```python
from build123d import *

# Parameters (mm, degrees)
SKETCH1_R               = 4.5
BOSS_EXTRUDE1_DEPTH     = 5
FILLET1_R               = 1
CUT_EXTRUDE1_DEPTH      = 78.139851996
CUT_EXTRUDE1_DEPTH_BACK = 78.139851996
CUT_EXTRUDE3_DEPTH      = 80.375373419
CUT_EXTRUDE3_DEPTH_BACK = 80.375373419


with BuildPart() as part:
    # Sketch1 → Boss-Extrude1 (new body)
    with BuildSketch(Plane.XY):
        with BuildLine():
            Line((-21.758850115, -29.16270467), (-30.758850115, -7.434782609))
            Line((-30.758850115, -7.434782609), (-30.758850115, 52.565217391))
            ThreePointArc((-30.758850115, 52.565217391), (-12.758850115, 70.565217391), (5.241149885, 52.565217391))
            Line((5.241149885, 52.565217391), (5.241149885, -7.434782609))
            Line((5.241149885, -7.434782609), (-3.758850115, -29.16270467))
            Line((-3.758850115, -29.16270467), (-12.758850115, -7.434782609))
            Line((-12.758850115, -7.434782609), (-21.758850115, -29.16270467))
        make_face()
        with Locations((-12.758850115, 52.565217391)):
            Circle(SKETCH1_R, mode=Mode.SUBTRACT)
    extrude(amount=BOSS_EXTRUDE1_DEPTH)

    # Fillet1
    fillet1_edges = [part.edges().sort_by_distance(p)[0] for p in [
        (5.241149885, 22.565217391, 5),
        (-17.258850115, 52.565217391, 0),
        (-17.258850115, 52.565217391, 5),
        (-12.758850115, 70.565217391, 5),
        (-30.758850115, 22.565217391, 5),
        (-30.758850115, 22.565217391, 0),
        (-12.758850115, 70.565217391, 0),
        (5.241149885, 22.565217391, 0),
    ]]
    fillet(fillet1_edges, radius=FILLET1_R)

    # Sketch5 → Cut-Extrude1 (cut, two sides: drawn at the far end of the back side and taken through both)
    with BuildSketch(Plane(origin=(0, 0, 0), x_dir=(0, 0, -1), z_dir=(1, 0, 0)).offset(-CUT_EXTRUDE1_DEPTH_BACK)):
        Polygon((-2.5, -29.16270467), (-5, -9.848996171), (-5, -29.16270467), align=None)
    extrude(amount=CUT_EXTRUDE1_DEPTH + CUT_EXTRUDE1_DEPTH_BACK, mode=Mode.SUBTRACT)

    # Sketch9 → Cut-Extrude3 (cut, two sides: drawn at the far end of the back side and taken through both)
    with BuildSketch(Plane(origin=(5.241149885, 0, 0), x_dir=(0, 0, -1), z_dir=(1, 0, 0)).offset(-CUT_EXTRUDE3_DEPTH_BACK)):
        Polygon((-2.5, -29.16270467), (0, -9.848996171), (0, -29.16270467), align=None)
    extrude(amount=CUT_EXTRUDE3_DEPTH + CUT_EXTRUDE3_DEPTH_BACK, mode=Mode.SUBTRACT)


solid = part.part
```
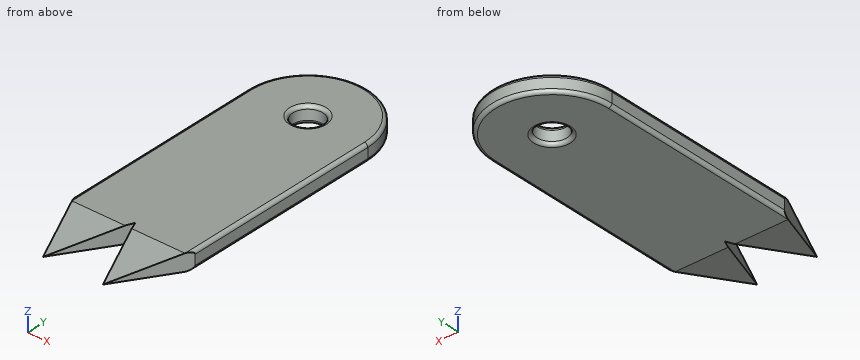
Here's how the part is built. I have some questions about the finished solid (model axes, mm). Give positions to 0.01 mm unless a question says otherwise; leave off trailing zeros. Loops run counter-clockwise (first coordinate to the right, second up) from the corner with the lowest first, then second, coordinate; pieces in that order, holes last. Notation, with made-up numbers: M 63,33 L 103,33 A34 ccw 103,63 Z; hole C -33,15 d6. An arc over 180 degrees is marked long. Use one line per item in the form item = value. Start each with the question number.
Q1. I need wall thicknesses on line 1 along X through (y, z) = (50.5, 2.3); line 2 along X through (y, z) = (51.5, 0.4); line 3 along Y through (x, z) = (0.5, 2.05). Which ranges of each line are inside material? Lowest first, please.
Q2. If we section it at A-A (y = -14): Write out the boundary of the cut face in (x, z).
Q3. Will these pins go through, and if not, where does the flat tip stop? pin 1 Ø1 at (x, z) = (1.5, 1.5) entering from -Y; pin 2 Ø8 at (x, y) = (-12.76, 52.57) entering from -Z.
Taken from the geometry:
q1.line_1 = -30.76 to -16.76, -8.76 to 5.24
q1.line_2 = -30.56 to -17.34, -8.18 to 5.04
q1.line_3 = -18.88 to 64.74
q2.outline = M -28.04,0.54 L -15.48,0.54 L -15.48,4.46 L -28.04,4.46 Z; M -10.04,0.54 L 2.52,0.54 L 2.52,4.46 L -10.04,4.46 Z
q3.pin_1 = -17.67
q3.pin_2 = through
